Verification items for the finished model (mm, model axes). Face numbers are marked on the shaded views. A direction names the side the tool comes from. Round coordinates to 2 decimals unless told otherwise and drop trailing zeros. Order: outer loops, then holes, each group sorted by start corner. A loop starts at its lowest first (then second) coordinate and runs counter-clockwise, first axis right, second up. Notation, with made-up numbers: (45, -40) -> (59, -40) arc R6 ccw to (59, -29) -> close; hole circle Ø4 at (30, -39). An arc over 180 degrees is marked (long way). Put each result on its own line as item: value.
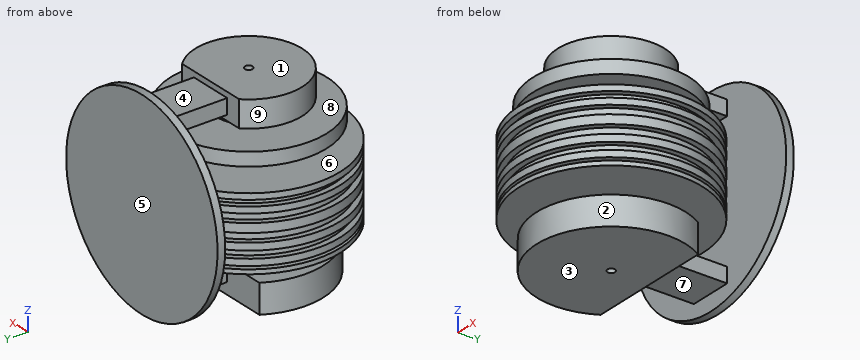
```python
from build123d import *

# Parameters (mm, degrees)
F2_W     = 95.933378
F2_H     = 103.010424
F3_DEPTH = 127
F4_W     = 72.550886
F4_H     = 25.166716
F5_DEPTH = 101.6
F6_R     = 165.1
F7_DEPTH = 12.7


with BuildPart() as f1:
    # F0 (on Front) → F1 (revolve)
    with BuildSketch(Plane.XZ):
        Polygon((88.794723, 147.411454), (6.476902, 147.411454), (6.476902, -157.388546), (123.8399, -157.388546), (123.8399, -109.347023), (31.267736, -109.347023), (31.267736, -80.914147), (152.272776, -80.914147), (152.272776, -73.552802), (142.721742, -73.552802), (142.721742, -68.588875), (152.272776, -68.588875), (152.272776, -57.600658), (142.721742, -57.600658), (142.721742, -45.443479), (152.272776, -45.443479), (152.272776, -33.520091), (142.721742, -33.520091), (142.721742, -19.024992), (152.272776, -19.024992), (152.272776, -4.062309), (142.721742, -4.062309), (142.721742, 10.198998), (152.272776, 10.198998), (152.272776, 20.719634), (142.721742, 20.719634), (142.721742, 30.772688), (152.272776, 30.772688), (152.272776, 40.75212), (31.267736, 40.75212), (31.267736, 68.523772), (129.790947, 68.523772), (129.790947, 91.005571), (53.749543, 91.005571), (53.749543, 103.568949), (88.794723, 103.568949), align=None)
    revolve(axis=Axis((0, 0, -4.988546), (0, 0, -1)))

    # F2 (on Right) → F3 (cut, symmetric)
    with BuildSketch(Plane.YZ):
        with Locations((111.389175, 147.290256)):
            Rectangle(F2_W, F2_H)
        Polygon((159.355864, -96.834429), (63.422486, -96.834429), (63.422486, -198.305756), (159.355864, -196.701795), align=None)
    extrude(amount=F3_DEPTH, both=True, mode=Mode.SUBTRACT)

    # F4 (on face) → F5 (join)
    with BuildSketch(Plane(origin=(0, 63.422486, 0), x_dir=(-1, 0, 0), z_dir=(0, 1, 0))):
        with Locations((0, 125.490201)):
            Rectangle(F4_W, F4_H)
        with Locations((0, -125.490201)):
            Rectangle(F4_W, F4_H)
    extrude(amount=F5_DEPTH)

    # F6 (on face) → F7 (join)
    with BuildSketch(Plane(origin=(0, 165.022486, 0), x_dir=(-1, 0, 0), z_dir=(0, 1, 0))):
        Circle(F6_R)
    extrude(amount=F7_DEPTH)


solid = f1.part
```
Item 1: Material ranges on line 1 along Y through (x, z) = (0, -67.5); line 2 along Y through (x, z) = (0, 80.5); line 3 along Z through (x, y) = (19.5, 90), recorded low to high.
Geometry check:
line 1: -152.27 to -6.48, 6.48 to 152.27, 165.02 to 177.72
line 2: -129.79 to -6.48, 6.48 to 129.79, 165.02 to 177.72
line 3: -138.07 to -112.91, -80.91 to 40.75, 68.52 to 91.01, 112.91 to 138.07
Item 2: Depth check by flat-ended pin: pin 1 Ø8 at (x, z) = (6, 130) entering from -Y; pin 2 Ø12 at (x, z) = (44, 132) entering from -Y; pin 3 Ø4 at (y, z) = (-5.5, -70.5) entering from +X. Enter the tip coordinate at first touch or a pass-through.
Geometry check:
pin 1: y = -88.77
pin 2: y = -80.25
pin 3: x = 152.19
Item 3: Sectioned sample at A-A, the plane x = 0. Give the number of separate pieces and of enclosed holes in the cut face, then the cut area to 3 significant figures.
Geometry check:
separate pieces: 2
enclosed holes: 1
area: 67,700 mm2
Item 4: Release check for a two-part mould opening along Z. For the marked faces 6, 7, 8 and 9 record: pulls with the +Z half, pulls with the -Z half, needs draft (parallel to the pull), parting line crosses it, or undercut.
Geometry check:
face 6: undercut
face 7: pulls with the -Z half
face 8: undercut
face 9: needs draft
Item 5: Sectioned sample at B-B, the plane z = -102.5. Record the boundary of the cut face in (x, y).
Geometry check:
outline: (-129.43, 165.02) -> (129.43, 165.02) -> (129.43, 177.72) -> (-129.43, 177.72) -> close; circle Ø62.54 at (0, 0); hole circle Ø12.95 at (0, 0)
Item 6: Tool access check on the marked faces 1, 2, 3, 4 and 5. Record the directions out of +Z, -Z, +X, -X, +Y, -Y that give a thin tool (end or side, any length) a straight path to the whole face; none if there is none.
Geometry check:
face 1: +Z, +X, -X, -Y
face 2: -Z
face 3: -Z, +X, -X, -Y
face 4: +Z, +X, -X
face 5: +Z, -Z, +X, -X, +Y
